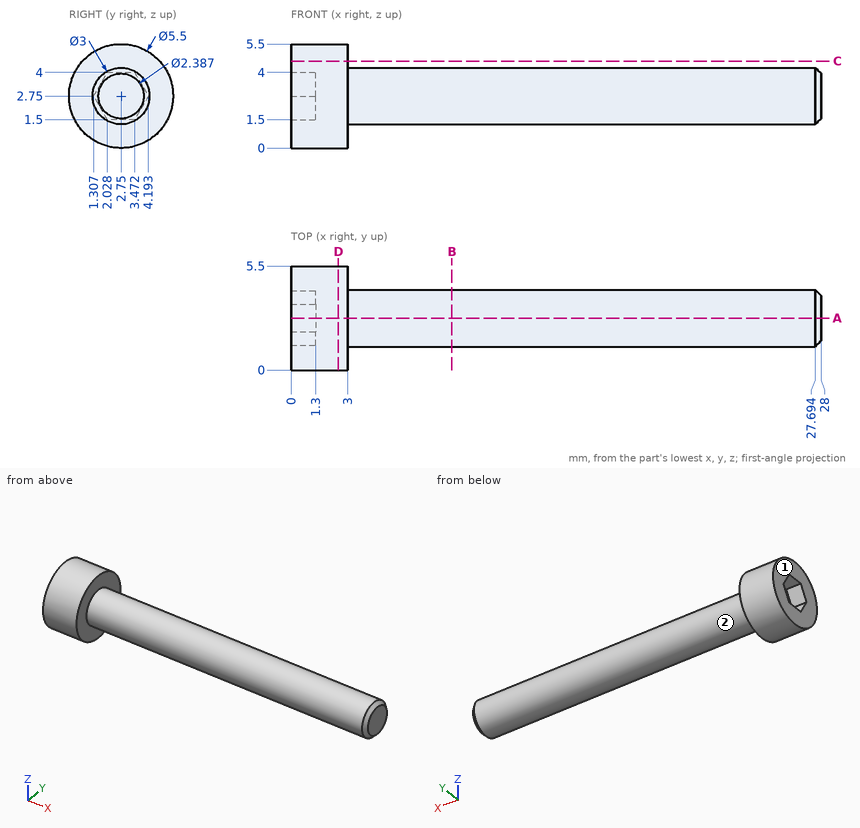
Design review of the part shown in the three views and the two pictorial views. Dimensions are in mm from the part's minimum x, y and z. A direction names the side the tool comes from. Round coordinates to 2 decimals unless told otherwise and drop trailing zeros. Loops run counter-clockwise (first coordinate to the right, second up) from the corner with the lowest first, then second, coordinate; pieces in that order, holes last. Notation, with made-up numbers: (41.5, 83.5) -> (58.5, 83.5) arc R18 ccw to (58.5, 88.5) -> close; hole circle Ø7 at (-34, -31). An arc over 180 degrees is marked (long way). Answer as a JSON object with one key per item and string values. Group by question number.
1) For pin 1 Ø1.5 at (x, z) = (3.5, 1) entering from -Y; pin 2 Ø2 at (x, z) = (7, 4.5) entering from -Y; pin 3 Ø1.5 at (x, z) = (19, 1) entering from +Y, all flat-tipped, find the tip position at first contact; note any pin that passes through.
2) We need section D-D on x = 2.5. Write out the cut boundary in (y, z).
3) For the marked faces 1 and 2, list the 3-axis set-ups (+Z, -Z, +X, -X, +Y, -Y) from which the entire face can be reached by the end or side of a thin tool; tool diameter is ignored.
4) We need section A-A on y = 2.75. Write out the cut boundary in (x, z).
5) We need section C-C on z = 4.6. Write out the cut boundary in (x, y) (1 decimal).
6) We need section B-B on x = 8.5. Write out the cut boundary in (y, z).
7) For line 1 (X direction, y = 4.05, z = 0.7); line 2 (X direction, y = 1.7, z = 2.45); line 3 (Y direction, x = 21.25, z = 3.65), list the stretches that pass through material, from the lowest coordinate up. Write a range as [from, to].
Result set:
{
 "1": {"pin 1": "y = 0.27", "pin 2": "y = 1.45", "pin 3": "y = 3.87"},
 "2": {"outline": "circle Ø5.5 at (2.75, 2.75)"},
 "3": {"face 1": "+Z, -Z, -X, +Y, -Y", "face 2": "+X"},
 "4": {"outline": "(0, 0) -> (3, 0) -> (3, 1.25) -> (27.69, 1.25) -> (28, 1.56) -> (28, 3.94) -> (27.69, 4.25) -> (3, 4.25) -> (3, 5.5) -> (0, 5.5) -> (0, 4) -> (1.3, 4) -> (1.3, 1.5) -> (0, 1.5) -> close"},
 "5": {"outline": "(0, 0.7) -> (3, 0.7) -> (3, 4.8) -> (0, 4.8) -> close"},
 "6": {"outline": "circle Ø3 at (2.75, 2.75)"},
 "7": {"line 1": "[0, 3]", "line 2": "[1.3, 28]", "line 3": "[1.55, 3.95]"}
}
